Answer from the drawing. Dimensions are ordinates in mm from the lowest x, y and z of the part. A direction names the side the tool comes from. Round coordinates to 2 decimals unless told otherwise and drop trailing zeros. Write each loop counter-clockwise with the first axis right and the second up, starting at its lowest first coordinate (ties: lowest second). Pieces come first, ordered by that corner, then holes. Notation, with made-up numbers: M -27,-3.75 L 31,-3.75 A19 ccw 31,31.25 Z; hole C 68,23 d11. An arc over 180 degrees is marked long. One line per item, written item: value. Start each with the question number.
(1) Section D-D (z = 1.1) is taken. Determine the outline of the cut face in (x, y), plus the area to 3 significant figures.
(2) Section B-B (z = 3.1) is taken. Determine the outline of the cut face in (x, y).
(3) Given P1, Ø1.5, axis at y = 17, z = 4.5, coming from the +X side; P2, Ø1, axis at x = 8, y = 11.5, coming from the +Z side; P3, Ø2.5, axis at y = 8.5, z = 2, coming from the +X side, each flat-ended and moving along its own axis, determine where each tip first touches the part or whether it passes through.
(4) For the marked faces 4 and 5, determine the directions among +Z, -Z, +X, -X, +Y, -Y from which every point of the face is accessible in a straight line to the end or side of a thin tool.
(5) For a pull along Y with two mould halves and no side action, classify the marked faces 1, 2 and 3 as released by +Y, released by -Y, zero draft, split by the parting line, or undercut.
(6) Section A-A (y = 14.91) is taken. Determine the outline of the cut face in (x, z).
(7) Section C-C (x = 3.65) is taken. Determine the outline of the cut face in (y, z), plus the area to 3 significant figures.
(8) Consider probe 1 along Y at (x, z) = (3.65, 1.15); probe 2 along X at (y, z) = (14.5, 3.7); probe 3 along X at (y, z) = (8.25, 1.65). Determine where each line is inside the solid, lowest interval first.
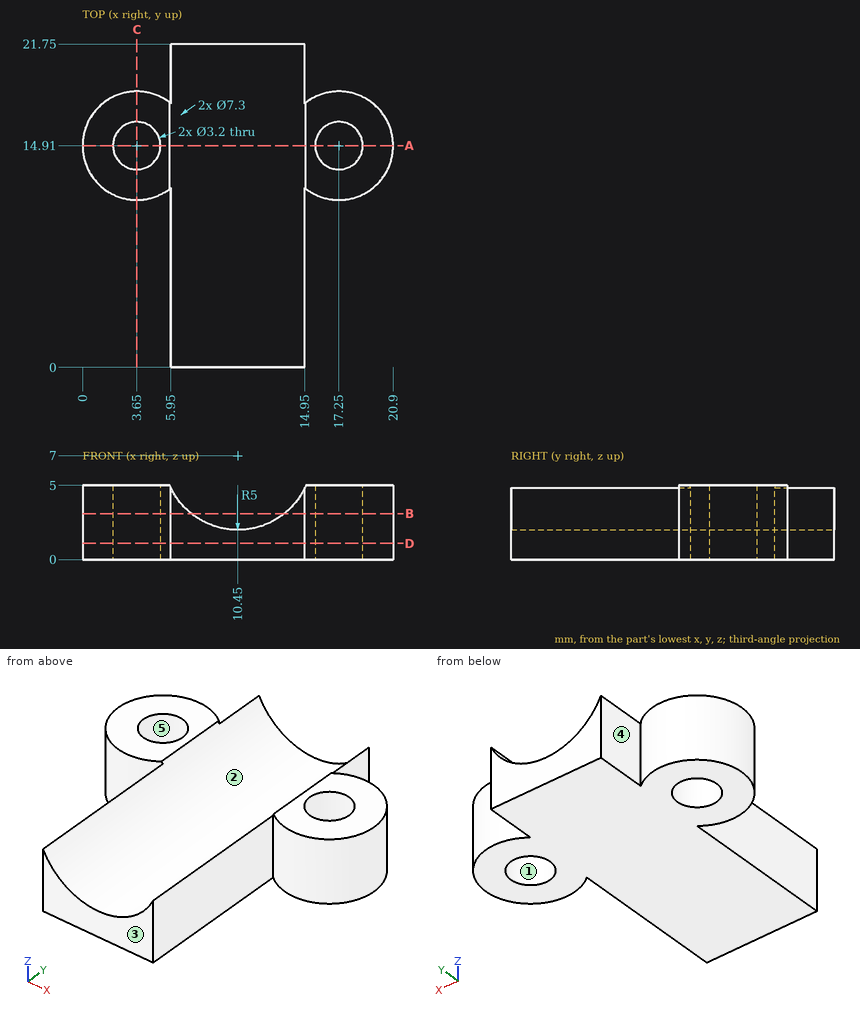
Recorded:
1. outline: M 5.95,0 L 14.95,0 L 14.95,12.08 A3.65 ccw long 14.95,17.74 L 14.95,21.75 L 5.95,21.75 L 5.95,17.74 A3.65 ccw long 5.95,12.08 Z; hole C 3.65,14.91 d3.2; hole C 17.25,14.91 d3.2
1. area: 253 mm2
2. outline: M 5.95,0 L 7.32,0 L 7.32,21.75 L 5.95,21.75 L 5.95,17.74 A3.65 ccw long 5.95,12.08 Z; M 13.58,0 L 14.95,0 L 14.95,12.08 A3.65 ccw long 14.95,17.74 L 14.95,21.75 L 13.58,21.75 Z; hole C 3.65,14.91 d3.2; hole C 17.25,14.91 d3.2
3. P1: stops at x = 20.65
3. P2: stops at z = 2.96
3. P3: stops at x = 14.95
4. face 4: +Z, -Z, +Y
4. face 5: +Z, -Z
5. face 1: undercut
5. face 2: zero draft
5. face 3: released by -Y
6. outline: M 0,0 L 2.05,0 L 2.05,5 L 0,5 Z; M 5.25,0 L 15.65,0 L 15.65,5 L 15.03,5 A5 cw 5.87,5 L 5.25,5 Z; M 18.85,0 L 20.9,0 L 20.9,5 L 18.85,5 Z
7. outline: M 11.26,0 L 13.31,0 L 13.31,5 L 11.26,5 Z; M 16.51,0 L 18.56,0 L 18.56,5 L 16.51,5 Z
7. area: 20.5 mm2
8. probe 1: y = 11.26 to 13.31, 16.51 to 18.56
8. probe 2: x = 0.02 to 2.1, 5.2 to 6.69, 14.21 to 15.7, 18.8 to 20.88
8. probe 3: x = 5.95 to 14.95
